Read the model definition and answer for the solid it produces. Units are mm, in the model's axes. A direction names the side the tool comes from. Round coordinates to 2 decimals unless told otherwise and drop trailing zeros. Order: outer loops, then holes, each group sorted by start corner. A loop starts at its lowest first (then second) coordinate and runs counter-clockwise, first axis right, second up. Notation, with made-up numbers: (79.5, 83.25) -> (125.5, 83.25) arc R6 cw to (125.5, 93.25) -> close; hole circle Ø4 at (75.25, 13). An arc over 180 degrees is marked (long way). Answer as a JSON object with one key per item and string values. Group by question number.
Item 1: Section B-B, the plane z = 11.75 is taken. Count the separate pieces of the cut face and the enclosed holes in it, plus the area to 3 significant figures.
Item 2: Section C-C, the plane y = 4 is taken. Write down the section's boundary in (x, z).
Item 3: Consider probe 1 along Y at (x, z) = (-12.5, 9.75); probe 2 along Y at (x, z) = (-22.8, 11.75); probe 3 along X at (y, z) = (-1, 13.5). Determine where each line is inside the solid, lowest interval first. Write a range as from..to.
Item 4: Section A-A, the plane x = -10 is taken. Write down the section's boundary in (y, z).
Item 5: Given P1, Ø4.5, axis at y = -8, z = 10, coming from the +X side; P2, Ø14, axis at x = 8, y = 26.5, coming from the +Z side; P3, Ø10, axis at y = 32.5, z = 4.5, coming from the +X side; P4, Ø7.5, axis at x = -11, y = 3.5, coming from the +Z side, each flat-ended and moving along its own axis, determine where each tip first touches the part or whether it passes through.
Item 6: For faces 4 (the flat face through (9.4, 33.7, 7.5)), 5 (the flat face through (-6.596, 6, 14)), 6 (the flat face through (-6.596, 31, 10)), 7 (the cylindrical face through (-23.37, 32.81, 12.69)), determine the directions among +Z, -Z, +X, -X, +Y, -Y from which every point of the face is accessible in a straight line to the end or side of a thin tool.
Item 7: The mould has two halves that part along Y. Classify faces 1 (the flat face through (-14, 6, 4.5)), 2 (the flat face through (-3.096, 13, 11)), 3 (the flat face through (0, 21.334, 4)): pulls with the +Y half, pulls with the -Y half, needs draft (parallel to the pull), parting line crosses it, or undercut.
Item 8: Section D-D, the plane z = 17.25 is taken. Write down the section's boundary in (x, y), plus the area to 3 significant figures.
from build123d import *

# Parameters (mm, degrees)
SKETCH1_W           = 22
SKETCH1_H           = 56
SKETCH1_W_2         = 15
SKETCH1_H_2         = 15
BOSS_EXTRUDE1_DEPTH = 20
SKETCH2_W           = 15
SKETCH2_H           = 15
SKETCH2_H_2         = 5.5
CUT_EXTRUDE1_DEPTH  = 15.5
SKETCH4_R           = 5.25
BOSS_EXTRUDE3_DEPTH = 7.5
FILLET4_R           = 1
SKETCH6_R           = 1.75
CUT_EXTRUDE2_DEPTH  = 10
CUT_EXTRUDE3_START  = -10
SKETCH7_R           = 1.75
CUT_EXTRUDE3_DEPTH  = 10


with BuildPart() as part:
    # Sketch1 → Boss-Extrude1 (new body)
    with BuildSketch(Plane.XY):
        with Locations((-14.096172604, 14.333947726)):
            Rectangle(SKETCH1_W, SKETCH1_H)
        with Locations((-14.096172604, 31.333947726)):
            Rectangle(SKETCH1_W_2, SKETCH1_H_2, mode=Mode.SUBTRACT)
    extrude(amount=BOSS_EXTRUDE1_DEPTH)

    # Sketch2 → Cut-Extrude1 (cut)
    with BuildSketch(Plane.XY.offset(20)):
        with Locations((-14.096172604, 6.333947726)):
            Rectangle(SKETCH2_W, SKETCH2_H)
        with Locations((-14.096172604, -7.416052274)):
            Rectangle(SKETCH2_W, SKETCH2_H_2)
    extrude(amount=-CUT_EXTRUDE1_DEPTH, mode=Mode.SUBTRACT)

    # Sketch4 → Boss-Extrude3 (add)
    with BuildSketch(Plane(origin=(0, 0, 0), x_dir=(-1, 0, 0), z_dir=(0, 0, -1))):
        with BuildLine():
            Line((-4.403827396, 41.333947726), (3.096172604, 41.333947726))
            Line((3.096172604, 41.333947726), (3.096172604, 21.333947726))
            Line((3.096172604, 21.333947726), (-4.403827396, 21.333947726))
            ThreePointArc((-4.403827396, 21.333947726), (-14.403827396, 31.333947726), (-4.403827396, 41.333947726))
        make_face()
        with Locations((-4.403827396, 31.333947726)):
            Circle(SKETCH4_R, mode=Mode.SUBTRACT)
    extrude(amount=-BOSS_EXTRUDE3_DEPTH)

    # Fillet4
    fillet4_edges = [part.edges().sort_by_distance(p)[0] for p in [
        (-3.096172604, 14.333947726, 20),
        (-25.096172604, 14.333947726, 0),
        (-25.096172604, 14.333947726, 20),
        (-14.096172604, 42.333947726, 20),
        (-3.096172604, 42.333947726, 10),
        (-14.096172604, 42.333947726, 0),
        (-25.096172604, 42.333947726, 10),
        (-3.096172604, 3.833947726, 0),
    ]]
    fillet(fillet4_edges, radius=FILLET4_R - 0.0001)  # a hair under: the kernel refuses the full size

    # Sketch6 → Cut-Extrude2 (cut)
    with BuildSketch(Plane.ZY.offset(25.096172604)):
        with Locations((11.75, 31.333947726)):
            Circle(SKETCH6_R)
        with Locations((11.75, 6.333947726)):
            Circle(SKETCH6_R)
    extrude(amount=-CUT_EXTRUDE2_DEPTH, mode=Mode.SUBTRACT)

    # Sketch7 → Cut-Extrude3 (cut)
    with BuildSketch(Plane(origin=(-3.096172604, 0, 0), x_dir=(0, 0, -1), z_dir=(1, 0, 0)).offset(CUT_EXTRUDE3_START)):
        with Locations(Location((-11.75, 6.333947726, 0), (0, 0, 180))):
            Circle(SKETCH7_R)
    extrude(amount=CUT_EXTRUDE3_DEPTH, mode=Mode.SUBTRACT)


solid = part.part
Values found:
{
 "1": {"separate pieces": "2", "enclosed holes": "1", "area": "662 mm2"},
 "2": {"outline": "(-25.1, 1) arc R1 ccw to (-24.1, 0) -> (-4.1, 0) arc R1 ccw to (-3.1, 1) -> (-3.1, 19) arc R1 ccw to (-4.1, 20) -> (-6.6, 20) -> (-6.6, 4.5) -> (-21.6, 4.5) -> (-21.6, 20) -> (-24.1, 20) arc R1 ccw to (-25.1, 19) -> close"},
 "3": {"probe 1": "-13.67..-10.17, -4.67..-1.17, 13.83..23.83, 38.83..42.33", "probe 2": "-13.67..4.58, 8.08..29.58, 33.08..42.33", "probe 3": "-25.1..-21.6, -6.6..-3.1"},
 "4": {"outline": "(-13.67, 0) -> (23.83, 0) -> (23.83, 20) -> (13.83, 20) -> (13.83, 4.5) -> (-1.17, 4.5) -> (-1.17, 20) -> (-4.67, 20) -> (-4.67, 4.5) -> (-10.17, 4.5) -> (-10.17, 20) -> (-13.67, 20) -> close; (38.83, 0) -> (41.33, 0) arc R1 ccw to (42.33, 1) -> (42.33, 19) arc R1 ccw to (41.33, 20) -> (38.83, 20) -> close"},
 "5": {"P1": "x = -3.1", "P2": "z = 7.5", "P3": "x = 14.4", "P4": "z = 4.5"},
 "6": {"face 4": "+Z, +X, +Y, -Y", "face 5": "+Z", "face 6": "+Z, -Z", "face 7": "-X"},
 "7": {"face 1": "undercut", "face 2": "needs draft", "face 3": "pulls with the -Y half"},
 "8": {"outline": "(-25.1, -13.67) -> (-3.1, -13.67) -> (-3.1, 41.33) arc R1 ccw to (-4.1, 42.33) -> (-24.1, 42.33) arc R1 ccw to (-25.1, 41.33) -> close; hole (-21.6, -10.17) -> (-6.6, -10.17) -> (-6.6, -4.67) -> (-21.6, -4.67) -> close; hole (-21.6, -1.17) -> (-6.6, -1.17) -> (-6.6, 13.83) -> (-21.6, 13.83) -> close; hole (-21.6, 23.83) -> (-6.6, 23.83) -> (-6.6, 38.83) -> (-21.6, 38.83) -> close", "area": "699 mm2"}
}
